```python
from build123d import *

# Parameters (mm, degrees)
F0_W     = 57.15
F0_H     = 22.86
F0_R     = 2.0955
F1_DEPTH = 9.398
F2_W     = 57.15
F2_H     = 2.5331471565
F3_DEPTH = 0.762
F4_W     = 57.15
F4_H     = 2.54
F5_DEPTH = 0.762
F6_SIZE  = 0.254


with BuildPart() as f1:
    # F0 (on Front) → F1 (new body)
    with BuildSketch(Plane.XZ):
        Rectangle(F0_W, F0_H)
        with Locations((-19.05, -1.905)):
            Circle(F0_R, mode=Mode.SUBTRACT)
        with Locations((19.05, -1.905)):
            Circle(F0_R, mode=Mode.SUBTRACT)
    extrude(amount=F1_DEPTH)

    # F2 (on face) → F3 (join)
    with BuildSketch(Plane(origin=(0, 0, 0), x_dir=(-1, 0, 0), z_dir=(0, 1, 0))):
        with Locations((0, -10.1634264217)):
            Rectangle(F2_W, F2_H)
    extrude(amount=F3_DEPTH)

    # F4 (on face) → F5 (join)
    with BuildSketch(Plane(origin=(0, 0, 0), x_dir=(-1, 0, 0), z_dir=(0, 1, 0))):
        with Locations((0, 10.16)):
            Rectangle(F4_W, F4_H)
    extrude(amount=F5_DEPTH)

    # F6
    f6_edges = [f1.edges().sort_by_distance(p)[0] for p in [
        (28.575, 0, -0.003426),
        (-28.575, -4.318, 11.43),
        (28.575, -4.318, 11.43),
        (0, 0.762, 11.43),
        (-21.1455, -9.398, -1.905),
        (16.9545, -9.398, -1.905),
        (0, -9.398, -11.43),
        (0, -9.398, 11.43),
        (28.575, -9.398, 0),
        (-28.575, -9.398, 0),
        (28.575, -4.318, -11.43),
        (-28.575, 0, -0.003426),
        (28.575, 0.762, 10.16),
        (28.575, 0.381, 8.89),
        (-28.575, -4.318, -11.43),
        (16.9545, 0, -1.905),
        (28.575, 0.381, -8.896853),
        (-21.1455, 0, -1.905),
        (28.575, 0.762, -10.163426),
        (0, 0.762, -11.43),
        (-28.575, 0.762, 10.16),
        (-28.575, 0.381, 8.89),
        (-28.575, 0.762, -10.163426),
        (-28.575, 0.381, -8.896853),
    ]]
    chamfer(f6_edges, length=F6_SIZE)


solid = f1.part
```
The listing builds one solid part. Answer for the finished solid, in the listing's coordinates (mm). A direction names the side the tool comes from. Round coordinates to 2 decimals unless told otherwise and drop trailing zeros. Loops run counter-clockwise (first coordinate to the right, second up) from the corner with the lowest first, then second, coordinate; pieces in that order, holes last.
Q1. Find the intervals of material crossed by line 1 (Z direction, x = 19.05, y = -4); line 2 (X direction, y = -2.5, z = -0.5) (3 decimals); line 3 (X direction, y = -7.75, z = -1.25) (1 decimal), in increasing order.
Q2. For a pull along Z with two mould halves and no side action, classify faces 1 (the face through (-20.713, -4.637, -3.18)), 2 (the face through (0, 0.762, 10)), 3 (the face through (0, -4, -11.43)) as released by +Z, released by -Z, zero draft, split by the parting line, or undercut.
Q3. Section C-C, the plane z = 4.75 is taken. Determine the outline of the cut face in (x, y) (3 decimals), then the cut area to 3 significant figures.
Q4. Given pin 1 Ø5 at (x, z) = (19.05, -1.905) entering from +Y, flat-ended and moving along its own axis, determine where the tip first touches the part or whether it passes through.
Q5. Which of the six approach directions +Z, -Z, +X, -X, +Y, -Y give full straight-line access (tool end or side, diameter ignored) to faces 4 (the face through (0, 0, 0)), 5 (the face through (21.05, -4.64, -1.28))?
Q6. Section B-B, the plane y = -6 is taken. Count the separate pieces of the cut face and the enclosed holes in it, then the cut area to 3 significant figures.
Q7. Section A-A, the plane x = -19.05 is taken. Determine the outline of the cut face in (y, z), then the cut area to 3 significant figures.
Q8. Section D-D, the plane x = -7.5 is taken. Determine the outline of the cut face in (y, z), then the cut area to 3 significant figures.
Completed:
1. line 1: z = -11.43 to -4, 0.19 to 11.43
1. line 2: x = -28.575 to -20.605, -17.495 to 17.495, 20.605 to 28.575
1. line 3: x = -28.6 to -21, -17.1 to 17.1, 21 to 28.6
2. face 1: undercut
2. face 2: zero draft
2. face 3: released by -Z
3. outline: (-28.575, -9.144) - (-28.321, -9.398) - (28.321, -9.398) - (28.575, -9.144) - (28.575, -0.254) - (28.321, 0) - (-28.321, 0) - (-28.575, -0.254) - close
3. area: 537 mm2
4. pin 1: stops at y = 0
5. face 4: +X, -X, +Y
5. face 5: +Y, -Y
6. separate pieces: 1
6. enclosed holes: 2
6. area: 1,280 mm2
7. outline: (-9.4, -11.18) - (-9.14, -11.43) - (0.51, -11.43) - (0.76, -11.18) - (0.76, -8.9) - (0, -8.9) - (0, -4.25) - (-0.25, -4) - (-9.14, -4) - (-9.4, -4.25) - close; (-9.4, 0.44) - (-9.14, 0.19) - (-0.25, 0.19) - (0, 0.44) - (0, 8.89) - (0.76, 8.89) - (0.76, 11.18) - (0.51, 11.43) - (-9.14, 11.43) - (-9.4, 11.18) - close
7. area: 179 mm2
8. outline: (-9.4, -11.18) - (-9.14, -11.43) - (0.51, -11.43) - (0.76, -11.18) - (0.76, -8.9) - (0, -8.9) - (0, 8.89) - (0.76, 8.89) - (0.76, 11.18) - (0.51, 11.43) - (-9.14, 11.43) - (-9.4, 11.18) - close
8. area: 219 mm2
